```python
from build123d import *

# Parameters (mm, degrees)
F0_W      = 90
F0_H      = 60
F1_DEPTH  = 5
F2_W      = 60
F2_H      = 40
F3_DEPTH  = 4
F4_R      = 5
F5_R      = 3
F7_R      = 3
F8_DEPTH  = 10
F9_R      = 3
F10_DEPTH = 7
F11_W     = 80
F11_H     = 50
F11_R     = 3
F12_DEPTH = 7
F13_R     = 3.75
F14_DEPTH = 5
F15_R     = 3.7177308685
F16_DEPTH = 5


with BuildPart() as f1:
    # F0 (on Top) → F1 (new body)
    with BuildSketch(Plane.XY):
        with Locations((0, -1.4884271659)):
            Rectangle(F0_W, F0_H)
    extrude(amount=F1_DEPTH)

    # F2 (on face) → F3 (join)
    with BuildSketch(Plane.XY.offset(5)):
        with Locations((0, -1.4884271659)):
            Rectangle(F2_W, F2_H)
    extrude(amount=F3_DEPTH)

    # F4
    f4_edges = [f1.edges().sort_by_distance(p)[0] for p in [
        (-45, 28.511573, 2.5),
        (45, 28.511573, 2.5),
        (45, -31.488427, 2.5),
        (-45, -31.488427, 2.5),
    ]]
    fillet(f4_edges, radius=F4_R)

    # F5
    f5_edges = [f1.edges().sort_by_distance(p)[0] for p in [
        (0, 28.511573, 5),
    ]]
    fillet(f5_edges, radius=F5_R)

    # F7 (on Top) → F8 (cut)
    with BuildSketch(Plane.XY):
        with Locations((-35.8441621065, 0)):
            Circle(F7_R)
        with Locations((36.2529978156, 0)):
            Circle(F7_R)
    extrude(amount=F8_DEPTH, mode=Mode.SUBTRACT)

    # F9 (on face) → F10 (join)
    with BuildSketch(Plane(origin=(0, 0, 0), x_dir=(1, 0, 0), z_dir=(0, 0, -1))):
        with BuildLine():
            ThreePointArc((40, -28.5115728341), (43.5355339059, -27.04710674), (45, -23.5115728341))
            Line((45, -23.5115728341), (45, 26.4884271659))
            ThreePointArc((45, 26.4884271659), (43.5355339059, 30.0239610718), (40, 31.4884271659))
            Line((40, 31.4884271659), (-40, 31.4884271659))
            ThreePointArc((-40, 31.4884271659), (-43.5355339059, 30.0239610718), (-45, 26.4884271659))
            Line((-45, 26.4884271659), (-45, -23.5115728341))
            ThreePointArc((-45, -23.5115728341), (-43.5355339059, -27.04710674), (-40, -28.5115728341))
            Line((-40, -28.5115728341), (40, -28.5115728341))
        make_face()
        with Locations((-35.8441621065, 0)):
            Circle(F9_R, mode=Mode.SUBTRACT)
        with Locations((36.2529978156, 0)):
            Circle(F9_R, mode=Mode.SUBTRACT)
    extrude(amount=F10_DEPTH)

    # F11 (on face) → F12 (cut)
    with BuildSketch(Plane(origin=(0, 0, -7), x_dir=(1, 0, 0), z_dir=(0, 0, -1))):
        with Locations((0, 1.4884271659)):
            Rectangle(F11_W, F11_H)
        with Locations((-35.8441621065, 0)):
            Circle(F11_R, mode=Mode.SUBTRACT)
        with Locations((36.2529978156, 0)):
            Circle(F11_R, mode=Mode.SUBTRACT)
    extrude(amount=-F12_DEPTH, mode=Mode.SUBTRACT)

    # F13 (on face) → F14 (join)
    with BuildSketch(Plane(origin=(0, 0, 0), x_dir=(1, 0, 0), z_dir=(0, 0, -1))):
        with Locations((-35.8441621065, 0)):
            Circle(F13_R)
    extrude(amount=F14_DEPTH)

    # F15 (on face) → F16 (join)
    with BuildSketch(Plane(origin=(0, 0, 0), x_dir=(1, 0, 0), z_dir=(0, 0, -1))):
        with Locations((36.2529978156, 0)):
            Circle(F15_R)
    extrude(amount=F16_DEPTH)


solid = f1.part
```
Work out the finished part from the listing and answer in its coordinate system (mm). A direction names the side the tool comes from. Coordinates: 2 decimals unless noted, no trailing zeros. Order: outer loops, then holes, each group sorted by start corner. A loop starts at its lowest first (then second) coordinate and runs counter-clockwise, first axis right, second up. Notation, with made-up numbers: (2, 29) - (23, 29) arc R28 ccw to (23, 60) - close; hole circle Ø9 at (-27, 37). An arc over 180 degrees is marked (long way). Answer as a JSON object with one key per item and string values.
1. A tool of negligible diameter and unlimited length cuts with its end or side. For faces 1 (the face through (0, -21.488, 7)), 2 (the face through (-30, -2, 7)), 3 (the face through (36, 0, 0)), 4 (the face through (30, -2, 7)), from which of +Z, -Z, +X, -X, +Y, -Y can it reach the whole face along a straight path? Write none if from no direction.
Output values:
{"face 1": "+Z, +X, -X, -Y", "face 2": "+Z, -X, +Y, -Y", "face 3": "+Z", "face 4": "+Z, +X, +Y, -Y"}
2. The mould has two halves that part along Y. Classify faces 5 (the face through (36, 0, -5)), 6 (the face through (44.1, -1.84, 4.14)), 7 (the face through (0.56, 27.609, 4.145)), 8 (the face through (-1, -2, 0)): +Y half, -Y half, draft (parallel to the pull), parting line (faces both ways), or undercut.
Output values:
{"face 5": "undercut", "face 6": "draft", "face 7": "+Y half", "face 8": "undercut"}
3. Find section B-B on x = -18.5. Determine the outline of the cut face in (y, z).
Output values:
{"outline": "(-31.49, -7) - (-26.49, -7) - (-26.49, 0) - (23.51, 0) - (23.51, -7) - (28.51, -7) - (28.51, 2) arc R3 ccw to (25.51, 5) - (18.51, 5) - (18.51, 9) - (-21.49, 9) - (-21.49, 5) - (-28.49, 5) arc R3 ccw to (-31.49, 2) - close"}
4. Each of these flat-tipped pins is pushed along its axis until it touches: P1, Ø6, axis at x = -34, y = 2, coming from the -Z side; P2, Ø4, axis at x = -30, y = 22.5, coming from the -Z side; P3, Ø6.5, axis at x = -37, y = 1, coming from the +Z side; P4, Ø4.5, axis at y = -4, z = 7, coming from the +X side. Where does it stop, or does it pass through?
Output values:
{"P1": "stops at z = -5", "P2": "stops at z = -7", "P3": "stops at z = 5", "P4": "stops at x = 43.2"}
5. Consider line 1 (X direction, y = 0, z = 1.3); line 2 (X direction, y = 0, z = 3.8); line 3 (Y direction, x = 39.5, z = -2.25). Determine where each line is inside the solid, lowest interval first.
Output values:
{"line 1": "x = -45 to -38.84, -32.84 to 33.25, 39.25 to 45", "line 2": "x = -44.4 to -38.84, -32.84 to 33.25, 39.25 to 44.4", "line 3": "y = -31.49 to -26.49, -1.81 to 1.81, 23.51 to 28.51"}
6. Find section D-D on y = -18. Determine the outline of the cut face in (x, z), plus the area to 3 significant figures.
Output values:
{"outline": "(-45, -7) - (-40, -7) - (-40, 0) - (40, 0) - (40, -7) - (45, -7) - (45, 2) arc R3 ccw to (42, 5) - (30, 5) - (30, 9) - (-30, 9) - (-30, 5) - (-42, 5) arc R3 ccw to (-45, 2) - close", "area": "756 mm²"}
7. Find section A-A on z = -1.25. Determine the outline of the cut face in (x, y).
Output values:
{"outline": "(-45, -26.49) arc R5 ccw to (-40, -31.49) - (40, -31.49) arc R5 ccw to (45, -26.49) - (45, 23.51) arc R5 ccw to (40, 28.51) - (-40, 28.51) arc R5 ccw to (-45, 23.51) - close; circle Ø7.5 at (-35.84, 0); circle Ø7.44 at (36.25, 0); hole (-40, -26.49) - (40, -26.49) - (40, 23.51) - (-40, 23.51) - close"}
